from build123d import *

# Parameters (mm, degrees)
SKETCH1_R           = 5
BOSS_EXTRUDE1_DEPTH = 6.2
CUT_EXTRUDE1_REACH  = 171.819
SKETCH2_R           = 2.5


with BuildPart() as part:
    # Sketch1 → Boss-Extrude1 (new body)
    with BuildSketch(Plane(origin=(0, 0, 0), x_dir=(1, 0, 0), z_dir=(0, 1, 0))):
        with BuildLine():
            Line((-15, -114.564392374), (-15, -98.868599666))
            ThreePointArc((-15, -98.868599666), (-70.710678119, -70.710678119), (-98.868599666, -15))
            Line((-98.868599666, -15), (-114.564392374, -15))
            ThreePointArc((-114.564392374, -15), (-117.942711997, -13.686048904), (-119.545452912, -10.434782609))
            ThreePointArc((-119.545452912, -10.434782609), (-120, 0), (-119.545452912, 10.434782609))
            ThreePointArc((-119.545452912, 10.434782609), (-117.942711997, 13.686048904), (-114.564392374, 15))
            Line((-114.564392374, 15), (-98.868599666, 15))
            ThreePointArc((-98.868599666, 15), (-70.710678119, 70.710678119), (-15, 98.868599666))
            Line((-15, 98.868599666), (-15, 114.564392374))
            ThreePointArc((-15, 114.564392374), (-13.686048904, 117.942711997), (-10.434782609, 119.545452912))
            ThreePointArc((-10.434782609, 119.545452912), (0, 120), (10.434782609, 119.545452912))
            ThreePointArc((10.434782609, 119.545452912), (13.686048904, 117.942711997), (15, 114.564392374))
            Line((15, 114.564392374), (15, 98.868599666))
            ThreePointArc((15, 98.868599666), (70.710678119, 70.710678119), (98.868599666, 15))
            Line((98.868599666, 15), (114.564392374, 15))
            ThreePointArc((114.564392374, 15), (117.942711997, 13.686048904), (119.545452912, 10.434782609))
            ThreePointArc((119.545452912, 10.434782609), (120, 0), (119.545452912, -10.434782609))
            ThreePointArc((119.545452912, -10.434782609), (117.942711997, -13.686048904), (114.564392374, -15))
            Line((114.564392374, -15), (98.868599666, -15))
            ThreePointArc((98.868599666, -15), (70.710678119, -70.710678119), (15, -98.868599666))
            Line((15, -98.868599666), (15, -114.564392374))
            ThreePointArc((15, -114.564392374), (13.686048904, -117.942711997), (10.434782609, -119.545452912))
            ThreePointArc((10.434782609, -119.545452912), (0, -120), (-10.434782609, -119.545452912))
            ThreePointArc((-10.434782609, -119.545452912), (-13.686048904, -117.942711997), (-15, -114.564392374))
        make_face()
        with Locations(Location((0, -110, 0), (0, 0, 270))):
            Circle(SKETCH1_R, mode=Mode.SUBTRACT)
        with Locations(Location((-110, 0, 0), (0, 0, 270))):
            Circle(SKETCH1_R, mode=Mode.SUBTRACT)
        with Locations(Location((0, 110, 0), (0, 0, 270))):
            Circle(SKETCH1_R, mode=Mode.SUBTRACT)
        with Locations(Location((110, 0, 0), (0, 0, 270))):
            Circle(SKETCH1_R, mode=Mode.SUBTRACT)
    extrude(amount=-BOSS_EXTRUDE1_DEPTH)

    # Sketch2 → Cut-Extrude1 (cut, up to next)
    with BuildSketch(Plane.XZ.offset(6.2), mode=Mode.PRIVATE) as cut_extrude1_sk1:
        with Locations(Location((18, 0, 0), (0, 0, 270))):
            Circle(SKETCH2_R)
    cut_extrude1_tool1 = extrude(cut_extrude1_sk1.sketch, amount=-CUT_EXTRUDE1_REACH, mode=Mode.PRIVATE) & part.part
    # Sketch2 → Cut-Extrude1 (cut, up to next)
    with BuildSketch(Plane.XZ.offset(6.2), mode=Mode.PRIVATE) as cut_extrude1_sk2:
        with Locations(Location((0, -18, 0), (0, 0, 270))):
            Circle(SKETCH2_R)
    cut_extrude1_tool2 = extrude(cut_extrude1_sk2.sketch, amount=-CUT_EXTRUDE1_REACH, mode=Mode.PRIVATE) & part.part
    # Sketch2 → Cut-Extrude1 (cut, up to next)
    with BuildSketch(Plane.XZ.offset(6.2), mode=Mode.PRIVATE) as cut_extrude1_sk3:
        with Locations(Location((-18, 0, 0), (0, 0, 270))):
            Circle(SKETCH2_R)
    cut_extrude1_tool3 = extrude(cut_extrude1_sk3.sketch, amount=-CUT_EXTRUDE1_REACH, mode=Mode.PRIVATE) & part.part
    # Sketch2 → Cut-Extrude1 (cut, up to next)
    with BuildSketch(Plane.XZ.offset(6.2), mode=Mode.PRIVATE) as cut_extrude1_sk4:
        with Locations(Location((0, 18, 0), (0, 0, 270))):
            Circle(SKETCH2_R)
    cut_extrude1_tool4 = extrude(cut_extrude1_sk4.sketch, amount=-CUT_EXTRUDE1_REACH, mode=Mode.PRIVATE) & part.part
    add(cut_extrude1_tool1.solids().sort_by_distance((18, -6.2, 0))[0], mode=Mode.SUBTRACT)
    add(cut_extrude1_tool2.solids().sort_by_distance((0, -6.2, -18))[0], mode=Mode.SUBTRACT)
    add(cut_extrude1_tool3.solids().sort_by_distance((-18, -6.2, 0))[0], mode=Mode.SUBTRACT)
    add(cut_extrude1_tool4.solids().sort_by_distance((0, -6.2, 18))[0], mode=Mode.SUBTRACT)


solid = part.part
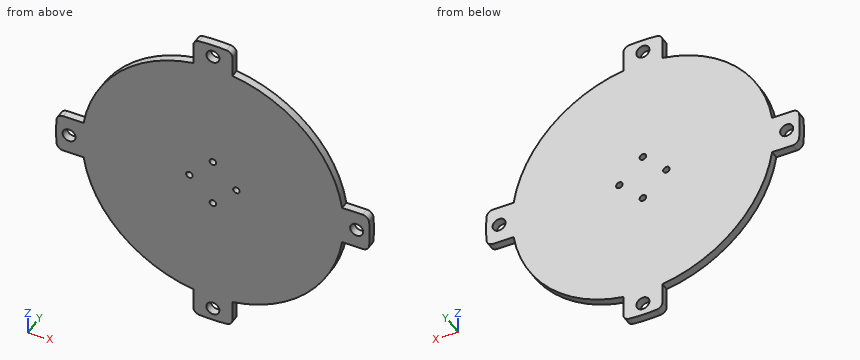
Could you check a few things on this model? Use its own coordinates, in mm. Coordinates: 2 decimals unless noted, no trailing zeros. Loops run counter-clockwise (first coordinate to the right, second up) from the corner with the lowest first, then second, coordinate; pieces in that order, holes last.
1. Imagine slicing it at D-D (z = 24.5). Please give me the cut outline in (x, y), and give its area (3 significant figures).
2. Imagine slicing it at C-C (y = -1.5). Give the number of separate pieces and of enclosed holes in the cut face, and give its area (3 significant figures).
3. I need wall thicknesses on L1, parallel to X at y = -3.5, z = 0; L2, parallel to X at y = -2.25, z = -110; L3, parallel to Z at x = -104, y = -4.75. Which ranges of each line are inside material? Lowest first, please.
4. Imagine slicing it at A-A (z = -110). Please give me the cut outline in (x, y), and give its area (3 significant figures).
5. For P1, Ø2, axis at x = 11, y = -1, coming from the -Z side; P2, Ø3, axis at x = 0, z = -18, coming from the -Y side; P3, Ø6, axis at x = 18, z = 0, coming from the -Y side; P4, Ø1.9, axis at y = -2, z = -110, coming from the -X side, each with a flat end and sliding along its axis, tell me the tip position at first contact or that it passes through.
6. Imagine slicing it at B-B (x = -110). Please give me the cut outline in (y, z), and give its area (3 significant figures).
Computed values:
1. outline: (-96.95, -6.2) - (96.95, -6.2) - (96.95, 0) - (-96.95, 0) - close
1. area: 1,200 mm2
2. separate pieces: 1
2. enclosed holes: 8
2. area: 33,400 mm2
3. L1: x = -120 to -115, -105 to -20.5, -15.5 to 15.5, 20.5 to 105, 115 to 120
3. L2: x = -15 to -5, 5 to 15
3. L3: z = -15 to 15
4. outline: (-15, -6.2) - (-5, -6.2) - (-5, 0) - (-15, 0) - close; (5, -6.2) - (15, -6.2) - (15, 0) - (5, 0) - close
4. area: 124 mm2
5. P1: stops at z = -119.58
5. P2: passes through
5. P3: stops at y = -6.2
5. P4: stops at x = -15
6. outline: (-6.2, -15) - (0, -15) - (0, -5) - (-6.2, -5) - close; (-6.2, 5) - (0, 5) - (0, 15) - (-6.2, 15) - close
6. area: 124 mm2
